Source: CAD feature listing. Evaluate the final solid. Frame: model axes, mm. A direction names the side the tool comes from. Give positions to 0.01 mm unless a question says otherwise; leave off trailing zeros. Loops run counter-clockwise (first coordinate to the right, second up) from the corner with the lowest first, then second, coordinate; pieces in that order, holes last. Notation, with made-up numbers: M 84,57 L 107,57 A31 ccw 107,83 Z; hole C -27,26 d5. An arc over 180 degrees is marked long. Answer in a Markdown table with one row per item.
```python
from build123d import *

# Parameters (mm, degrees)
SKETCH1_R           = 60.625
SKETCH1_R_2         = 45
BOSS_EXTRUDE1_DEPTH = 4
SKETCH2_R           = 49
SKETCH2_R_2         = 45
BOSS_EXTRUDE2_DEPTH = 45
SKETCH3_R           = 45
BOSS_EXTRUDE3_DEPTH = 4
BOSS_EXTRUDE7_START = 2
SKETCH4_R           = 60.625
SKETCH4_R_2         = 56.502019499
SKETCH4_R_3         = 46.502019499
BOSS_EXTRUDE7_DEPTH = 2
SKETCH5_R           = 2.5
SKETCH5_R_2         = 2
CUT_EXTRUDE1_DEPTH  = 10
SKETCH6_W           = 11
SKETCH6_H           = 5
CUT_EXTRUDE2_DEPTH  = 10


with BuildPart() as part:
    # Sketch1 → Boss-Extrude1 (new body)
    with BuildSketch(Plane(origin=(0, 0, 0), x_dir=(1, 0, 0), z_dir=(0, 1, 0))):
        with Locations(Location((-5.233283161, 2.275340505, 0), (0, 0, 270))):
            Circle(SKETCH1_R)
        with Locations(Location((-5.233283161, 2.275340505, 0), (0, 0, 270))):
            Circle(SKETCH1_R_2, mode=Mode.SUBTRACT)
    extrude(amount=BOSS_EXTRUDE1_DEPTH)

    # Sketch2 → Boss-Extrude2 (add)
    with BuildSketch(Plane(origin=(0, 4, 0), x_dir=(1, 0, 0), z_dir=(0, 1, 0))):
        with Locations(Location((-5.233283161, 2.275340505, 0), (0, 0, 90))):
            Circle(SKETCH2_R)
        with Locations(Location((-5.233283161, 2.275340505, 0), (0, 0, 270))):
            Circle(SKETCH2_R_2, mode=Mode.SUBTRACT)
    extrude(amount=BOSS_EXTRUDE2_DEPTH)

    # Sketch3 → Boss-Extrude3 (add)
    with BuildSketch(Plane(origin=(0, 0, 0), x_dir=(-1, 0, 0), z_dir=(0, -1, 0))):
        with Locations(Location((5.233283161, 2.275340505, 0), (0, 0, 90))):
            Circle(SKETCH3_R)
    extrude(amount=-BOSS_EXTRUDE3_DEPTH)

    # Sketch4 → Boss-Extrude7 (add)
    # profile 1 of 2: a face of its own
    with BuildSketch(Plane.XZ.offset(BOSS_EXTRUDE7_START)):
        with Locations(Location((-5.233283161, -2.275340505, 0), (0, 0, 270))):
            Circle(SKETCH4_R)
        with Locations(Location((-5.233283161, -2.275340505, 0), (0, 0, 270))):
            Circle(SKETCH4_R_2, mode=Mode.SUBTRACT)
    # profile 2 of 2: a face of its own
    with BuildSketch(Plane.XZ.offset(BOSS_EXTRUDE7_START)):
        with Locations(Location((-5.233283161, -2.275340505, 0), (0, 0, 90))):
            Circle(SKETCH4_R_3)
    extrude(amount=-BOSS_EXTRUDE7_DEPTH)

    # Sketch5 → Cut-Extrude1 (cut)
    with BuildSketch(Plane(origin=(0, -2, 0), x_dir=(-1, 0, 0), z_dir=(0, -1, 0))):
        with Locations(Location((5.233283161, 2.275340505, 0), (0, 0, 90))):
            Circle(SKETCH5_R)
        with Locations(Location((-10.766716839, -13.724659495, 0), (0, 0, 90))):
            Circle(SKETCH5_R_2)
        with Locations(Location((21.233283161, -13.724659495, 0), (0, 0, 90))):
            Circle(SKETCH5_R_2)
        with Locations(Location((21.233283161, 18.275340505, 0), (0, 0, 90))):
            Circle(SKETCH5_R_2)
        with Locations(Location((-10.766716839, 18.275340505, 0), (0, 0, 90))):
            Circle(SKETCH5_R_2)
    extrude(amount=-CUT_EXTRUDE1_DEPTH, mode=Mode.SUBTRACT)

    # Sketch6 → Cut-Extrude2 (cut)
    with BuildSketch(Plane(origin=(43.766716839, 0, 0), x_dir=(0, 0, -1), z_dir=(1, 0, 0))):
        with Locations((0.504292548, 42.858395169)):
            Rectangle(SKETCH6_W, SKETCH6_H)
    extrude(amount=-CUT_EXTRUDE2_DEPTH, mode=Mode.SUBTRACT)


solid = part.part
```
1) Pin query (flat end, axial travel): pin 1 Ø4 at (x, z) = (-4, -22.5) entering from +Y; pin 2 Ø1 at (y, z) = (6.5, -44.5) entering from -X; pin 3 Ø4 at (y, z) = (20, -6.5) entering from -X. Return the tip coordinate at first contact, or that it passes through.
Reply:
| item | result |
|---|---|
| pin 1 | stops at y = 4 |
| pin 2 | stops at x = -30.92 |
| pin 3 | stops at x = -54.18 |
2) Section A-A, the plane z = 26.5. Return loops of the section in (x, y), then the cut area to 3 significant figures.
Reply:
| item | result |
|---|---|
| outline | M -58.59,-2 L -53.86,-2 L -53.86,0 L -41.76,0 L -41.76,-2 L 31.3,-2 L 31.3,0 L 43.39,0 L 43.39,-2 L 48.13,-2 L 48.13,4 L 34.43,4 L 34.43,49 L 29.36,49 L 29.36,4 L -39.83,4 L -39.83,49 L -44.89,49 L -44.89,4 L -58.59,4 Z |
| area | 1,050 mm² |
3) Material intervals for L1, parallel to X at y = 16.5, z = -3; L2, parallel to Y at x = 8, z = -56; L3, parallel to Y at x = 5, z = -50, sorted ascending.
Reply:
| item | result |
|---|---|
| L1 | x = -54.23 to -50.23, 39.76 to 43.76 |
| L2 | y = 0 to 4 |
| L3 | y = 0 to 49 |
4) Pull-direction query (Y, two-part tool) for faces 1 (the flat face through (4, -2, -3)), 2 (the flat face through (42, 45.358, 0)), 3 (the cylindrical face through (8.814, 0.958, 14.158)), 4 (the flat face through (-15, 4, -2)); classes: released by +Y, released by -Y, zero draft, split by the parting line, or undercut.
Reply:
| item | result |
|---|---|
| face 1 | released by -Y |
| face 2 | undercut |
| face 3 | zero draft |
| face 4 | released by +Y |
5) Section B-B, the plane x = -26. Return loops of the section in (y, z), then the cut area to 3 significant figures.
Reply:
| item | result |
|---|---|
| outline | M -2,-59.23 L 4,-59.23 L 4,-46.66 L 49,-46.66 L 49,-42.2 L 4,-42.2 L 4,37.65 L 49,37.65 L 49,42.11 L 4,42.11 L 4,54.68 L -2,54.68 L -2,50.27 L 0,50.27 L 0,39.33 L -2,39.33 L -2,-43.88 L 0,-43.88 L 0,-54.82 L -2,-54.82 Z |
| area | 1,040 mm² |
6) Section C-C, the plane y = 13. Return loops of the section in (x, z).
Reply:
| item | result |
|---|---|
| outline | C -5.23,-2.28 d98; hole C -5.23,-2.28 d90 |
7) Set-up query: faces 5 (the flat face through (-13, 0, 44)), 6 (the flat face through (34.5, 49, -23.8)), 7 (the cylindrical face through (42.6, 26.18, 8.35)), 8 (the flat face through (42, 40.358, 0)). Return all of +Z, -Z, +X, -X, +Y, -Y with unobstructed straight access to the full face (end or side cutting, diameter ignored); none if empty.
Reply:
| item | result |
|---|---|
| face 5 | -Y |
| face 6 | +Z, -Z, +X, -X, +Y |
| face 7 | +Y |
| face 8 | +X |
